Read the model definition and answer for the solid it produces. Units are mm, in the model's axes. Face numbers are marked on the shaded views. A direction names the side the tool comes from. Coordinates: 2 decimals unless noted, no trailing zeros. Write each loop counter-clockwise with the first axis right and the second up, starting at its lowest first coordinate (ties: lowest second). Pieces come first, ordered by that corner, then holes. Notation, with made-up numbers: (37.5, 80.25) -> (47.5, 80.25) arc R25 cw to (47.5, 104.25) -> close; hole circle Ø7 at (-3, 10.25). An arc over 180 degrees is marked (long way). Answer in a Markdown table with one row per item. Add a question column.
Item 1: For a pull along X with two mould halves and no side action, classify the marked faces 1, 2 and 3 as +X half, -X half, draft (parallel to the pull), parting line (faces both ways), or undercut.
Item 2: Section C-C on x = 2 is taken. Write down the section's boundary in (y, z), then the cut area to 3 significant figures.
Item 3: Which of the six approach directions +Z, -Z, +X, -X, +Y, -Y give full straight-line access (tool end or side, diameter ignored) to the marked faces 4, 5 and 6?
Item 4: Section B-B on z = 9.5 is taken. Write down the section's boundary in (x, y).
Item 5: Given pin 1 Ø10 at (x, z) = (-1, 14.5) entering from -Y; pin 2 Ø6 at (y, z) = (-43, 7) entering from -X; pin 3 Ø6 at (y, z) = (-41.5, 11) entering from +X, each flat-ended and moving along its own axis, determine where each tip first touches the part or whether it passes through.
Item 6: Section A-A on y = -48 is taken. Write down the section's boundary in (x, z).
Item 7: Straight lines are drawn through the part: line 1 (X direction, y = -33, z = 4.75); line 2 (Y direction, x = 7, z = 12.25). For each, find the intervals that lie inside material, in ascending order. Write a range as from..to.
Solid Edge part; units mm, degrees
sketch "Sketch1" plane through (0, 0, 0) normal (0, 0, 1) x (1, 0, 0)
  line L0 (-41.5811, -19.5976) -> (38.4189, -19.5976)
  line L1 (38.4189, -19.5976) -> (38.4189, 20.4024)
  line L2 (38.4189, 20.4024) -> (-41.5811, 20.4024)
  line L3 (-41.5811, 20.4024) -> (-41.5811, -19.5976)
extrude "Protrusion1" add sketch "Sketch1" along normal blind 20
sketch "Sketch2" plane through (-1.5811, -19.5976, 10) normal (0, -1, 0) x (1, 0, 0)
  line L0 (-20, 10) -> (-20, -10)
  line L1 (-20, -10) -> (-10, -10)
  line L2 (-10, -10) -> (-10, 10)
  line L3 (-10, 10) -> (-20, 10)
  line L4 (20, 10) -> (20, -10)
  line L5 (20, -10) -> (10, -10)
  line L6 (10, -10) -> (10, 10)
  line L7 (10, 10) -> (20, 10)
extrude "ExtrudedProtrusion_2" add sketch "Sketch2" along normal blind 50
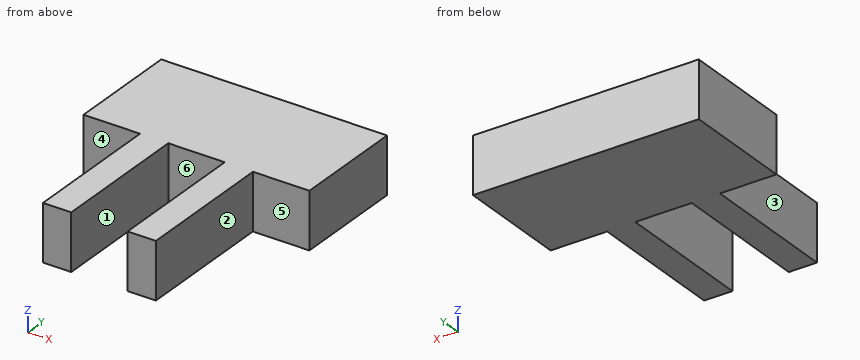
Results below:
| question | item | result |
|---|---|---|
| 1 | face 1 | undercut |
| 1 | face 2 | +X half |
| 1 | face 3 | -X half |
| 2 | outline | (-19.6, 0) -> (20.4, 0) -> (20.4, 20) -> (-19.6, 20) -> close |
| 2 | area | 800 mm2 |
| 3 | face 4 | +Z, -Z, -X, -Y |
| 3 | face 5 | +Z, -Z, +X, -Y |
| 3 | face 6 | +Z, -Z, -Y |
| 4 | outline | (-41.58, -19.6) -> (-21.58, -19.6) -> (-21.58, -69.6) -> (-11.58, -69.6) -> (-11.58, -19.6) -> (8.42, -19.6) -> (8.42, -69.6) -> (18.42, -69.6) -> (18.42, -19.6) -> (38.42, -19.6) -> (38.42, 20.4) -> (-41.58, 20.4) -> close |
| 5 | pin 1 | stops at y = -19.6 |
| 5 | pin 2 | stops at x = -21.58 |
| 5 | pin 3 | stops at x = 18.42 |
| 6 | outline | (-21.58, 0) -> (-11.58, 0) -> (-11.58, 20) -> (-21.58, 20) -> close; (8.42, 0) -> (18.42, 0) -> (18.42, 20) -> (8.42, 20) -> close |
| 7 | line 1 | x = -21.58..-11.58, 8.42..18.42 |
| 7 | line 2 | y = -19.6..20.4 |
